Check sheet for the modelled part. Datum: model origin and axes. Units: mm. A direction names the side the tool comes from. Round coordinates to 2 decimals unless told otherwise and drop trailing zeros. Write each loop counter-clockwise with the first axis right and the second up, starting at its lowest first coordinate (ties: lowest second). Pieces come first, ordered by that corner, then holes. Notation, with made-up numbers: (1, 34.25) -> (35, 34.25) arc R30 ccw to (35, 67.25) -> close; hole circle Ø3 at (25.5, 71). An arc over 180 degrees is marked (long way). One line per item, written item: value.
Autodesk Inventor part; units mm, degrees
ref_plane "YZ Plane" through (0, 0, 0) normal (1, 0, 0) x (0, 1, 0)
ref_plane "XZ Plane" through (0, 0, 0) normal (0, 1, 0) x (-1, 0, 0)
ref_plane "XY Plane" through (0, 0, 0) normal (0, 0, 1) x (1, 0, 0)
sketch "Sketch2" plane through (0, 0, 0) normal (0, 0, 1) x (1, 0, 0)
  line L0 (0, 0) -> (8, 0)
  line L1 (8, 0) -> (8, 8)
  line L2 (8, 8) -> (0, 8)
  line L3 (0, 8) -> (0, 0)
  point P0 (4, 4)
  dimension "d2" = 8
  dimension "d3" = 8
extrude "Extrusion1" add sketch "Sketch2" along normal blind 10
sketch "Sketch3" plane through (0, 0, 10) normal (0, 0, 1) x (1, 0, 0)
  point P0 (0, 0)
  point P1 (4, 4)
hole "Hole1" at (4, 4, 10) direction (0, 0, -1) diameter 3.2 depth 10 counterbore diameter 4.1 counterbore depth 0.6
fillet "Fillet1" radius 2 4 edges at (8, 8, 5) (0, 8, 5) (8, 0, 5) (0, 0, 5)
properties part number "Insert Test"
Item 1: Depth check by flat-ended pin: pin 1 (4.5 mm diameter, centred on x = 4.5, y = 4, fed in from +Z); pin 2 (1.9 mm diameter, centred on x = 4, y = 4, fed in from -Z). Enter the tip coordinate at first touch or a pass-through.
Result set:
pin 1: z = 10
pin 2: through
Item 2: Sectioned sample at C-C (z = 7.5). Enter the section's corners in (x, y).
Result set:
outline: (0, 2) arc R2 ccw to (2, 0) -> (6, 0) arc R2 ccw to (8, 2) -> (8, 6) arc R2 ccw to (6, 8) -> (2, 8) arc R2 ccw to (0, 6) -> close; hole circle Ø3.2 at (4, 4)
Item 3: Sectioned sample at A-A (y = 4). Enter the section's corners in (x, z).
Result set:
outline: (0, 0) -> (2.4, 0) -> (2.4, 9.4) -> (1.95, 9.4) -> (1.95, 10) -> (0, 10) -> close; (5.6, 0) -> (8, 0) -> (8, 10) -> (6.05, 10) -> (6.05, 9.4) -> (5.6, 9.4) -> close
Item 4: Material ranges on line 1 along X through (y, z) = (4, 9.9); line 2 along Y through (x, z) = (4, 7), recorded low to high.
Result set:
line 1: 0 to 1.95, 6.05 to 8
line 2: 0 to 2.4, 5.6 to 8
Item 5: Sectioned sample at D-D (x = 2.25). Enter the section's corners in (y, z).
Result set:
outline: (0, 0) -> (8, 0) -> (8, 10) -> (5.07, 10) -> (5.07, 9.4) -> (2.93, 9.4) -> (2.93, 10) -> (0, 10) -> close
Item 6: Tool access check on faces 1 (the flat face through (4, 0, 5)), 2 (the cylindrical face through (3.91, 6.05, 9.7)). Record the directions out of +Z, -Z, +X, -X, +Y, -Y that give a thin tool (end or side, any length) a straight path to the whole face; none if there is none.
Result set:
face 1: +Z, -Z, +X, -X, -Y
face 2: +Z
Item 7: Release check for a two-part mould opening along Y. For faces 3 (the cylindrical face through (2.92, 5.18, 4.63)), 4 (the flat face through (3, 6, 10)), 5 (the cylindrical face through (0.57, 0.6, 5.07)), 6 (the cylindrical face through (7.43, 7.4, 5.07)) record: pulls with the +Y half, pulls with the -Y half, needs draft (parallel to the pull), parting line crosses it, or undercut.
Result set:
face 3: undercut
face 4: needs draft
face 5: pulls with the -Y half
face 6: pulls with the +Y half
